from build123d import *

# Parameters (mm, degrees)
SKETCH1_R           = 38.5
BOSS_EXTRUDE1_DEPTH = 115
SKETCH2_R           = 2.6
BOSS_EXTRUDE2_DEPTH = 5
SKETCH3_R           = 38.5
SKETCH3_R_2         = 30.3
BOSS_EXTRUDE3_DEPTH = 2
FILLET1_R           = 1


with BuildPart() as part:
    # Sketch1 → Boss-Extrude1 (new body)
    with BuildSketch(Plane(origin=(0, 0, 0), x_dir=(1, 0, 0), z_dir=(0, 1, 0))):
        with Locations(Location((0, 0, 0), (0, 0, 270))):
            Circle(SKETCH1_R)
    extrude(amount=BOSS_EXTRUDE1_DEPTH)

    # Sketch2 → Boss-Extrude2 (add)
    # profile 1 of 2: a face of its own
    with BuildSketch(Plane(origin=(0, 115, 0), x_dir=(1, 0, 0), z_dir=(0, 1, 0))):
        with BuildLine():
            Line((-21.25, 4.153311931), (-21.25, -4.153311931))
            ThreePointArc((-21.25, -4.153311931), (-16.25, -6.5), (-11.25, -4.153311931))
            Line((-11.25, -4.153311931), (-11.25, 4.153311931))
            ThreePointArc((-11.25, 4.153311931), (-16.25, 6.5), (-21.25, 4.153311931))
        make_face()
        with Locations(Location((-16.25, 0, 0), (0, 0, 270))):
            Circle(SKETCH2_R, mode=Mode.SUBTRACT)
    # profile 2 of 2: a face of its own
    with BuildSketch(Plane(origin=(0, 115, 0), x_dir=(1, 0, 0), z_dir=(0, 1, 0))):
        with BuildLine():
            Line((12.096688069, 5), (20.403311931, 5))
            ThreePointArc((20.403311931, 5), (22.75, 0), (20.403311931, -5))
            Line((20.403311931, -5), (12.096688069, -5))
            ThreePointArc((12.096688069, -5), (9.75, 0), (12.096688069, 5))
        make_face()
        with Locations(Location((16.25, 0, 0), (0, 0, 270))):
            Circle(SKETCH2_R, mode=Mode.SUBTRACT)
    extrude(amount=BOSS_EXTRUDE2_DEPTH)

    # Sketch3 → Boss-Extrude3 (add)
    with BuildSketch(Plane(origin=(0, 115, 0), x_dir=(1, 0, 0), z_dir=(0, 1, 0))):
        with Locations(Location((0, 0, 0), (0, 0, 270))):
            Circle(SKETCH3_R)
        with Locations(Location((0, 0, 0), (0, 0, 270))):
            Circle(SKETCH3_R_2, mode=Mode.SUBTRACT)
    extrude(amount=BOSS_EXTRUDE3_DEPTH)

    # Fillet1
    fillet1_edges = [part.edges().sort_by_distance(p)[0] for p in [
        (0, 0, -38.5),
        (0, 117, -38.5),
    ]]
    fillet(fillet1_edges, radius=FILLET1_R)


solid = part.part
Work out the finished part from the listing and answer in its coordinate system (mm). A direction names the side the tool comes from. Give positions to 0.01 mm unless a question says otherwise; leave off trailing zeros. Order: outer loops, then holes, each group sorted by start corner. A loop starts at its lowest first (then second) coordinate and runs counter-clockwise, first axis right, second up. Notation, with made-up numbers: (-28.5, 23) - (5.5, 23) arc R30 ccw to (5.5, 51) - close; hole circle Ø9 at (27, 3). An arc over 180 degrees is marked (long way). Answer as CSV lines item,"result". Start each with the question number.
Q1. For faces 1 (the face through (16, 117, -5)), 2 (the face through (-19, 120, -2)), determine the directions among +Z, -Z, +X, -X, +Y, -Y from which every point of the face is accessible in a straight line to the end or side of a thin tool.
Q2. The part is cut by section B-B (z = 0). Write down the section's boundary in (x, y), then the cut area to 3 significant figures.
Q3. The mould has two halves that part along X. Classify faces 3 (the face through (-37.584, 57.695, -8.346)), 4 (the face through (-21.25, 117, 0)), 5 (the face through (-30.4, 117, -3)): +X half, -X half, draft (parallel to the pull), parting line (faces both ways), or undercut.
Q4. Find the intervals of material crossed by L1, parallel to X at y = 116, z = 0; L2, parallel to X at y = 117.1, z = 0; L3, parallel to X at y = 116.8, z = 0, in increasing order. Write a range as [from, to].
Q5. The part is cut by section C-C (y = 87.5). Write down the section's boundary in (x, z), then the cut area to 3 significant figures.
Q6. Given pin 1 Ø1.5 at (y, z) = (105.5, -2.5) entering from +X; pin 2 Ø3 at (x, y) = (8, 54) entering from -Z; pin 3 Ø4 at (x, z) = (15.5, 0.5) entering from +Y; pin 4 Ø2 at (x, y) = (3, 37) entering from -Z, each flat-ended and moving along its own axis, determine where each tip first touches the part or whether it passes through.
Q7. The part is cut by section A-A (x = 0). Write down the section's boundary in (y, z), then the cut area to 3 significant figures.
Check result:
1,face 1,"+Y"
1,face 2,"+Z, -Z, +X, -X, +Y"
2,outline,"(-38.5, 1) arc R1 ccw to (-37.5, 0) - (37.5, 0) arc R1 ccw to (38.5, 1) - (38.5, 116) arc R1 ccw to (37.5, 117) - (30.3, 117) - (30.3, 115) - (22.75, 115) - (22.75, 120) - (18.85, 120) - (18.85, 115) - (13.65, 115) - (13.65, 120) - (9.75, 120) - (9.75, 115) - (-11.25, 115) - (-11.25, 120) - (-13.65, 120) - (-13.65, 115) - (-18.85, 115) - (-18.85, 120) - (-21.25, 120) - (-21.25, 115) - (-30.3, 115) - (-30.3, 117) - (-37.5, 117) arc R1 ccw to (-38.5, 116) - close"
2,area,"8,950 mm²"
3,face 3,"parting line"
3,face 4,"undercut"
3,face 5,"draft"
4,L1,"x = [-38.5, -30.3], [-21.25, -18.85], [-13.65, -11.25], [9.75, 13.65], [18.85, 22.75], [30.3, 38.5]"
4,L2,"x = [-21.25, -18.85], [-13.65, -11.25], [9.75, 13.65], [18.85, 22.75]"
4,L3,"x = [-38.1, -30.3], [-21.25, -18.85], [-13.65, -11.25], [9.75, 13.65], [18.85, 22.75], [30.3, 38.1]"
5,outline,"circle Ø77 at (0, 0)"
5,area,"4,660 mm²"
6,pin 1,"stops at x = 38.46"
6,pin 2,"stops at z = -37.95"
6,pin 3,"stops at y = 120"
6,pin 4,"stops at z = -38.45"
7,outline,"(0, -37.5) arc R1 ccw to (1, -38.5) - (116, -38.5) arc R1 ccw to (117, -37.5) - (117, -30.3) - (115, -30.3) - (115, 30.3) - (117, 30.3) - (117, 37.5) arc R1 ccw to (116, 38.5) - (1, 38.5) arc R1 ccw to (0, 37.5) - close"
7,area,"8,890 mm²"
